Here's the drawing with two shaded views (mm, measured from the low corner). I have some questions. Coordinates: 2 decimals unless noted, no trailing zeros. Write each loop counter-clockwise with the first axis right and the second up, starting at its lowest first coordinate (ties: lowest second). Pieces come first, ordered by that corner, then holes. Notation, with made-up numbers: (62.5, 42) -> (70.5, 42) arc R29 ccw to (70.5, 72) -> close; hole circle Ø2 at (37, 31.25). An arc over 180 degrees is marked (long way). Put each result on its own line as item: value.
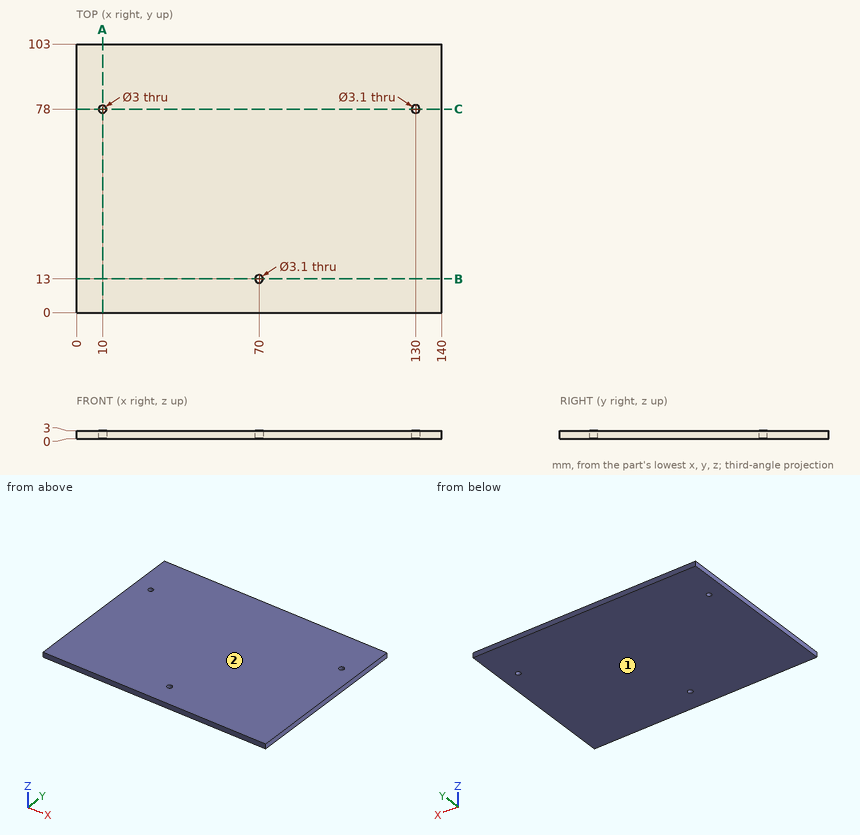
Item 1: For P1, Ø3, axis at x = 70, y = 13, coming from the -Z side, with a flat end and sliding along its axis, tell me the tip position at first contact or that it passes through.
Output:
P1: passes through
Item 2: Please list where these lines run through material, in increasing order: line 1 along X through (y, z) = (78, 0.7); line 2 along Y through (x, z) = (130, 1.25); line 3 along Y through (x, z) = (70, 0.7). Write a range as from..to.
Output:
line 1: x = 0..8.5, 11.5..128.45, 131.55..140
line 2: y = 0..76.45, 79.55..103
line 3: y = 0..11.45, 14.55..103
Item 3: Imagine slicing it at C-C on y = 78. Write out the boundary of the cut face in (x, z).
Output:
outline: (0, 0) -> (8.5, 0) -> (8.5, 3) -> (0, 3) -> close; (11.5, 0) -> (128.45, 0) -> (128.45, 3) -> (11.5, 3) -> close; (131.55, 0) -> (140, 0) -> (140, 3) -> (131.55, 3) -> close
Item 4: Imagine slicing it at A-A on x = 10. Write out the boundary of the cut face in (y, z), then the cut area to 3 significant figures.
Output:
outline: (0, 0) -> (76.5, 0) -> (76.5, 3) -> (0, 3) -> close; (79.5, 0) -> (103, 0) -> (103, 3) -> (79.5, 3) -> close
area: 300 mm²
Item 5: If we mould it in two halves opening along Z, with no side actions, what happens to the marked faces 1 and 2? For each: released by +Z, released by -Z, zero draft, split by the parting line, or undercut.
Output:
face 1: released by -Z
face 2: released by +Z
Item 6: Imagine slicing it at B-B on y = 13. Write out the boundary of the cut face in (x, z), then the cut area to 3 significant figures.
Output:
outline: (0, 0) -> (68.45, 0) -> (68.45, 3) -> (0, 3) -> close; (71.55, 0) -> (140, 0) -> (140, 3) -> (71.55, 3) -> close
area: 411 mm²
